Input: dimensioned drawing with shaded views. Units: mm. Origin: part minimum x, y, z. Give positions to 0.01 mm unless a question says otherwise; leave off trailing zeros. Order: outer loops, then holes, each group sorted by start corner. A loop starts at its lowest first (then second) coordinate and runs counter-clockwise, first axis right, second up. Notation, with made-up numbers: M -39,6.25 L -11,6.25 A8 ccw -11,15.25 Z; hole C 31,-4 d2. An arc over 180 degrees is marked long. Answer in a Markdown table with one row per item. Add a question column.
(1) Mould query, pull axis X, two halves, no side actions, for the marked faces 1, 2 and 3. Classes: pulls with the +X half, pulls with the -X half, needs draft (parallel to the pull), parting line crosses it, or undercut.
(2) Section query C-C, the plane z = 11.5. Return loops of the section in (x, y).
(3) Section query D-D, the plane x = 50.5. Return loops of the section in (y, z).
(4) Section query A-A, the plane y = 81.28. Return loops of the section in (x, z), plus the area to 3 significant figures.
(5) Section query B-B, the plane x = 31.75. Return loops of the section in (y, z), plus the area to 3 significant figures.
(6) Material intervals for line 1 along Y through (x, z) = (51, 1) (1 decimal); line 2 along Y through (x, z) = (31.75, 9.25); line 3 along Y through (x, z) = (52.07, 5.75), sorted ascending.
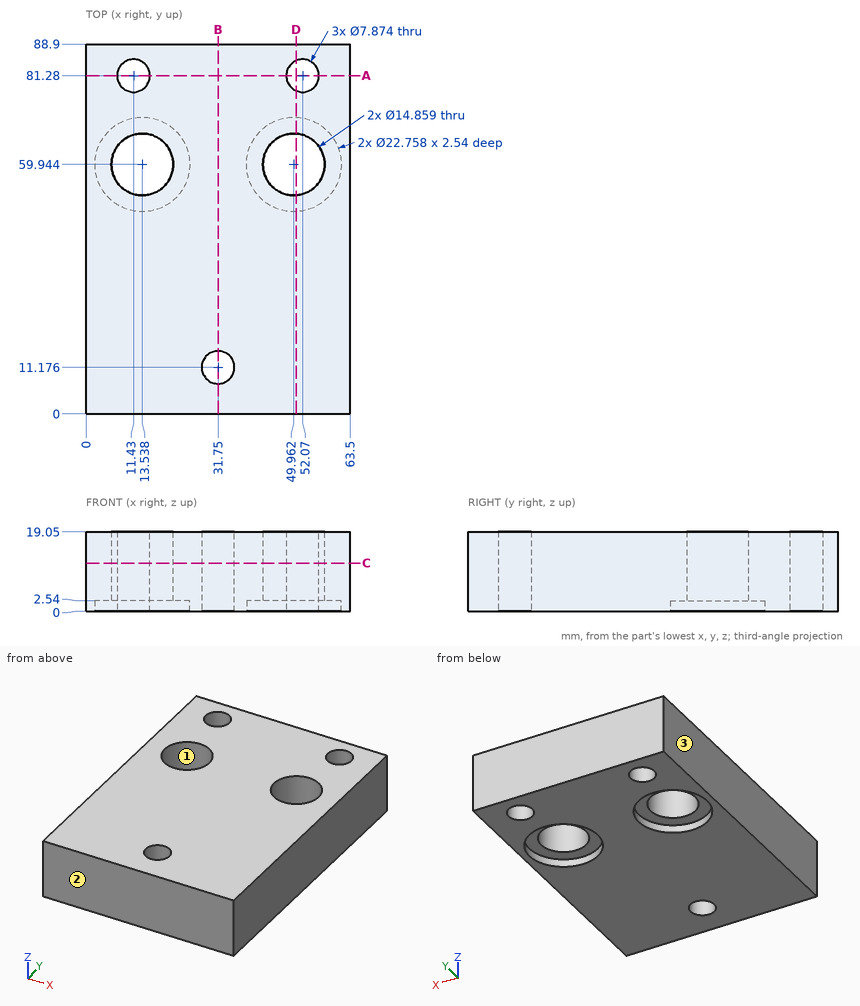
Values follow:
| question | item | result |
|---|---|---|
| 1 | face 1 | undercut |
| 1 | face 2 | needs draft |
| 1 | face 3 | pulls with the -X half |
| 2 | outline | M 0,0 L 63.5,0 L 63.5,88.9 L 0,88.9 Z; hole C 13.54,59.94 d14.86; hole C 11.43,81.28 d7.87; hole C 31.75,11.18 d7.87; hole C 49.96,59.94 d14.86; hole C 52.07,81.28 d7.87 |
| 3 | outline | M 0,0 L 48.58,0 L 48.58,2.54 L 52.53,2.54 L 52.53,19.05 L 0,19.05 Z; M 67.35,2.54 L 71.31,2.54 L 71.31,0 L 77.67,0 L 77.67,19.05 L 67.35,19.05 Z; M 84.89,0 L 88.9,0 L 88.9,19.05 L 84.89,19.05 Z |
| 4 | outline | M 0,0 L 7.49,0 L 7.49,19.05 L 0,19.05 Z; M 15.37,0 L 48.13,0 L 48.13,19.05 L 15.37,19.05 Z; M 56.01,0 L 63.5,0 L 63.5,19.05 L 56.01,19.05 Z |
| 4 | area | 910 mm² |
| 5 | outline | M 0,0 L 7.24,0 L 7.24,19.05 L 0,19.05 Z; M 15.11,0 L 88.9,0 L 88.9,19.05 L 15.11,19.05 Z |
| 5 | area | 1,540 mm² |
| 6 | line 1 | y = 0 to 48.6, 71.3 to 77.5, 85.1 to 88.9 |
| 6 | line 2 | y = 0 to 7.24, 15.11 to 88.9 |
| 6 | line 3 | y = 0 to 52.82, 67.07 to 77.34, 85.22 to 88.9 |
